Could you check a few things on this model? Use its own coordinates, in mm. A direction names the side the tool comes from. Coordinates: 2 decimals unless noted, no trailing zeros. Loops run counter-clockwise (first coordinate to the right, second up) from the corner with the lowest first, then second, coordinate; pieces in that order, holes last.
from build123d import *

# Parameters (mm, degrees)
SKETCH1_W           = 79.8
SKETCH1_H           = 79.8
BOSS_EXTRUDE1_DEPTH = 9.6
SKETCH3_W           = 93.857769302
SKETCH3_H           = 7.7
SKETCH3_W_2         = 31.7
SKETCH3_H_2         = 31.7
SKETCH3_W_3         = 95.7
SKETCH3_H_3         = 7.8
SKETCH3_W_4         = 7.8
SKETCH3_H_4         = 95.7
BOSS_EXTRUDE2_DEPTH = 19.3


with BuildPart() as part:
    # Sketch1 → Boss-Extrude1 (new body)
    with BuildSketch(Plane(origin=(0, 0, 0), x_dir=(1, 0, 0), z_dir=(0, 1, 0))):
        with Locations((-0.532, -4.965333333)):
            Rectangle(SKETCH1_W, SKETCH1_H)
    extrude(amount=BOSS_EXTRUDE1_DEPTH)

    # Sketch3 → Boss-Extrude2 (add)
    with BuildSketch(Plane.XZ):
        with Locations((0.389115349, 16.965333333)):
            Rectangle(SKETCH3_W, SKETCH3_H)
        with Locations((-0.532, 4.965333333)):
            Rectangle(SKETCH3_W_2, SKETCH3_H_2)
        with Locations((-0.532, -6.984666667)):
            Rectangle(SKETCH3_W_3, SKETCH3_H_3)
        with Locations((-12.482, 4.965333333)):
            Rectangle(SKETCH3_W_4, SKETCH3_H_4)
        with Locations((11.418, 4.965333333)):
            Rectangle(SKETCH3_W_4, SKETCH3_H_4)
    extrude(amount=BOSS_EXTRUDE2_DEPTH)


solid = part.part
(1) Imagine slicing it at A-A, the plane x = 41. Write out the boundary of the cut face in (y, z).
Answers:
outline: (-19.3, -10.88) - (0, -10.88) - (0, -3.08) - (-19.3, -3.08) - close; (-19.3, 13.12) - (0, 13.12) - (0, 20.82) - (-19.3, 20.82) - close
(2) Imagine slicing it at B-B, the plane x = -12.5. Write out the boundary of the cut face in (y, z), and give its area (3 significant figures).
Answers:
outline: (-19.3, -42.88) - (0, -42.88) - (0, -34.93) - (9.6, -34.93) - (9.6, 44.87) - (0, 44.87) - (0, 52.82) - (-19.3, 52.82) - close
area: 2,610 mm2
(3) Which directions (+Z, -Z, +X, -X, +Y, -Y) give clear straight access to the entire face, cutting with the end or side of a thin tool? Please do faces 1 (the face through (7.518, -10, 37)), 2 (the face through (43, 0, -7)), 3 (the face through (7.518, -10, -27)), 4 (the face through (11, 0, 49)), 5 (the face through (-40.432, 5, 6)).
Answers:
face 1: +Z, -Y
face 2: +Z, -Z, +X, +Y
face 3: -Z, -Y
face 4: +Z, +X, -X, +Y
face 5: +Z, -Z, -X, +Y
(4) Imagine slicing it at D-D, the plane z = -1.5. Write out the boundary of the cut face in (x, y).
Answers:
outline: (-40.43, 0) - (-16.38, 0) - (-16.38, -19.3) - (15.32, -19.3) - (15.32, 0) - (39.37, 0) - (39.37, 9.6) - (-40.43, 9.6) - close
(5) For pin 1 (3 mm diameter, centred on y = -13.5, z = 34.5, fed in from +X); pin 2 (9.5 mm diameter, centred on y = -10, z = -27, fed in from -X); pin 3 (6 mm diameter, centred on x = 14, y = 4, fed in from +Z), each with a flat end and sliding along its axis, tell me the tip position at first contact or that it passes through.
Answers:
pin 1: stops at x = 15.32
pin 2: stops at x = -16.38
pin 3: stops at z = 44.87
(6) We'd pull the mould along Z, two halves only. Please class faces 6 (the face through (32, -10, 20.815)), 7 (the face through (-33, -10, -3.085)), 8 (the face through (27, 0, 5)), 9 (the face through (-33, -10, -10.885)): +Z half, -Z half, draft (parallel to the pull), parting line (faces both ways), or undercut.
Answers:
face 6: +Z half
face 7: undercut
face 8: undercut
face 9: -Z half
(7) Imagine slicing it at C-C, the plane y = -10.75. Write out the boundary of the cut face in (x, z), and give its area (3 significant figures).
Answers:
outline: (-48.38, -10.88) - (-16.38, -10.88) - (-16.38, -42.88) - (-8.58, -42.88) - (-8.58, -10.88) - (7.52, -10.88) - (7.52, -42.88) - (15.32, -42.88) - (15.32, -10.88) - (47.32, -10.88) - (47.32, -3.08) - (15.32, -3.08) - (15.32, 13.12) - (47.32, 13.12) - (47.32, 20.82) - (15.32, 20.82) - (15.32, 52.82) - (7.52, 52.82) - (7.52, 20.82) - (-8.58, 20.82) - (-8.58, 52.82) - (-16.38, 52.82) - (-16.38, 20.82) - (-46.54, 20.82) - (-46.54, 13.12) - (-16.38, 13.12) - (-16.38, -3.08) - (-48.38, -3.08) - close
area: 2,980 mm2
(8) I need wall thicknesses on probe 1 along Z at (x, y) = (-28, -8.5); probe 2 along X at (y, z) = (-16.5, 26.5); probe 3 along Z at (x, y) = (-27, 8). Which ranges of each line are inside material? Lowest first, please.
Answers:
probe 1: z = -10.88 to -3.08, 13.12 to 20.82
probe 2: x = -16.38 to -8.58, 7.52 to 15.32
probe 3: z = -34.93 to 44.87
